Geometry: see drawing. Coordinates: mm, zero at the bounding-box minimum. Give positions to 0.01 mm unless a question says otherwise; leave off trailing zeros. Loops run counter-clockwise (first coordinate to the right, second up) from the corner with the lowest first, then second, coordinate; pieces in that order, holes last. Notation, with made-up numbers: M -28,86.5 L -5,86.5 A21 ccw -5,120.5 Z; hole C 76,85.5 d6. An arc over 180 degrees is marked long. Answer in a Markdown table with one row per item.
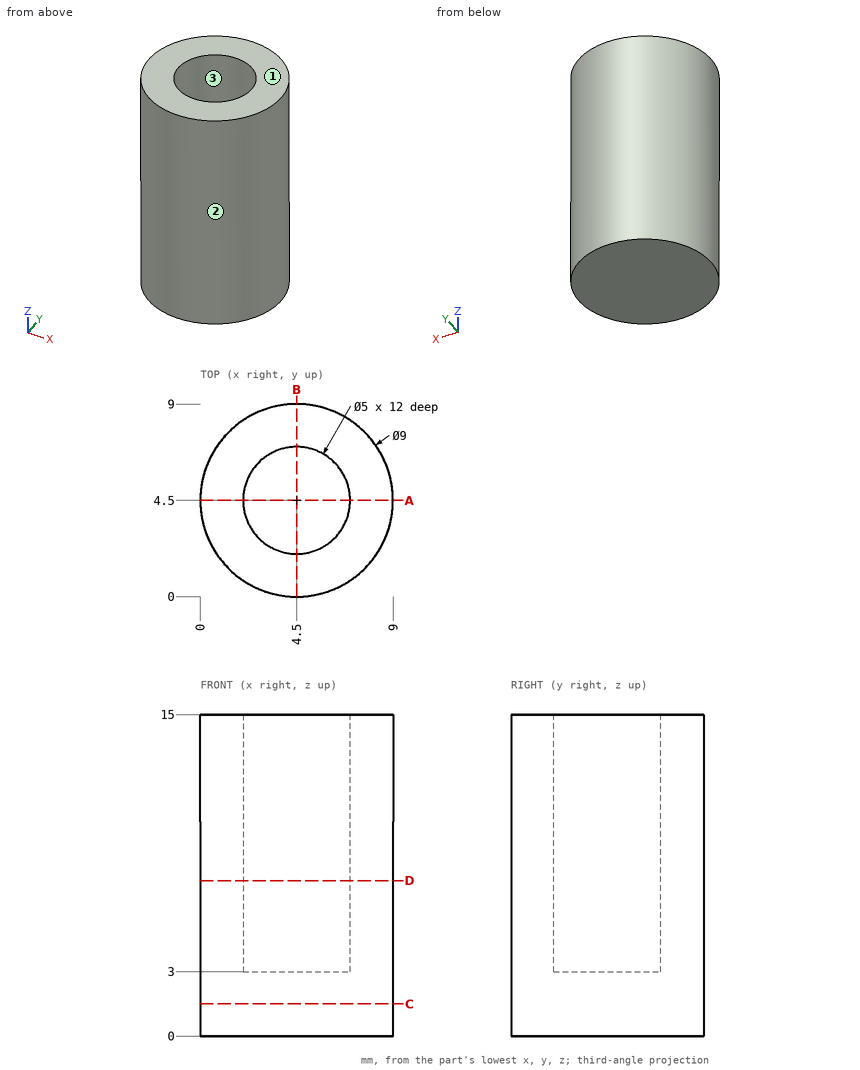
1) Material intervals for L1, parallel to Y at x = 4.5, z = 10.25; L2, parallel to Z at x = 3.5, y = 6, sorted ascending.
Reply:
| item | result |
|---|---|
| L1 | y = 0 to 2, 7 to 9 |
| L2 | z = 0 to 3 |
2) Pull-direction query (X, two-part tool) for the marked faces 1, 2 and 3; classes: released by +X, released by -X, zero draft, split by the parting line, or undercut.
Reply:
| item | result |
|---|---|
| face 1 | zero draft |
| face 2 | split by the parting line |
| face 3 | undercut |
3) Pin query (flat end, axial travel): pin 1 Ø1 at (x, z) = (6.5, 3.5) entering from -Y; pin 2 Ø1.5 at (y, z) = (7, 1.5) entering from -X; pin 3 Ø4 at (x, y) = (4.5, 4.5) entering from +Z. Return the tip coordinate at first contact, or that it passes through.
Reply:
| item | result |
|---|---|
| pin 1 | stops at y = 0.26 |
| pin 2 | stops at x = 0.35 |
| pin 3 | stops at z = 3 |
4) Section D-D, the plane z = 7.25. Return loops of the section in (x, y).
Reply:
| item | result |
|---|---|
| outline | C 4.5,4.5 d9; hole C 4.5,4.5 d5 |
5) Section A-A, the plane y = 4.5. Return loops of the section in (x, z).
Reply:
| item | result |
|---|---|
| outline | M 0,0 L 9,0 L 9,15 L 7,15 L 7,3 L 2,3 L 2,15 L 0,15 Z |
6) Section C-C, the plane z = 1.5. Return loops of the section in (x, y), then the cut area to 3 significant figures.
Reply:
| item | result |
|---|---|
| outline | C 4.5,4.5 d9 |
| area | 63.6 mm² |
